For this review, take the finished solid that the model builds, in its own axes (mm). Give positions to 0.01 mm unless a question says otherwise; leave off trailing zeros. Loops run counter-clockwise (first coordinate to the right, second up) from the corner with the lowest first, then second, coordinate; pieces in that order, holes last. Notation, with made-up numbers: (57.25, 41) - (103.25, 41) arc R23 cw to (103.25, 75) - close; hole circle Ø2 at (-14, 15). An arc over 180 degrees is marked (long way). Answer in a Markdown table with one row per item.
```python
from build123d import *

# Parameters (mm, degrees)
CROQUIS1_W              = 50
CROQUIS1_H              = 55
CROQUIS1_R              = 3
SALIENTE_EXTRUIR1_DEPTH = 2.9
REDONDEO1_R             = 2
REDONDEO2_R             = 2


with BuildPart() as part:
    # Croquis1 → Saliente-Extruir1 (new body)
    with BuildSketch(Plane.XY):
        with Locations((25, 27.5)):
            Rectangle(CROQUIS1_W, CROQUIS1_H)
        with Locations((30, 42.5)):
            Circle(CROQUIS1_R, mode=Mode.SUBTRACT)
    extrude(amount=SALIENTE_EXTRUIR1_DEPTH)

    # Redondeo1
    redondeo1_edges = [part.edges().sort_by_distance(p)[0] for p in [
        (50, 0, 1.45),
        (0, 0, 1.45),
    ]]
    fillet(redondeo1_edges, radius=REDONDEO1_R)

    # Redondeo2
    redondeo2_edges = [part.edges().sort_by_distance(p)[0] for p in [
        (0, 55, 1.45),
        (50, 55, 1.45),
    ]]
    fillet(redondeo2_edges, radius=REDONDEO2_R)


solid = part.part
```
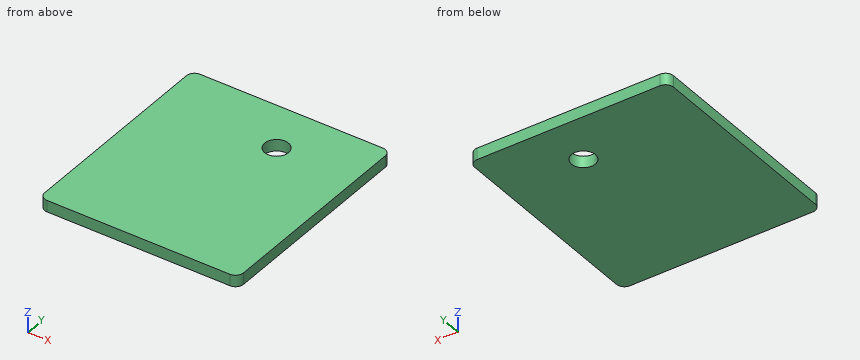
1. Clearance check with a flat-ended pin moving along its axis: pin 1 (3.5 mm diameter, centred on x = 30, y = 42.5, fed in from +Z). State where the tip first meets the part, or that it passes through.
Values:
| item | result |
|---|---|
| pin 1 | passes through |
2. Wall thickness on line 1 (Y direction, x = 30, z = 2.3): over which ranges is the line inside the solid? List them lowest first. Write a range as [from, to].
Values:
| item | result |
|---|---|
| line 1 | y = [0, 39.5], [45.5, 55] |
3. We need section A-A, the plane y = 42.5. Give the boundary of the cut face in (x, z), and give its area (3 significant figures).
Values:
| item | result |
|---|---|
| outline | (0, 0) - (27, 0) - (27, 2.9) - (0, 2.9) - close; (33, 0) - (50, 0) - (50, 2.9) - (33, 2.9) - close |
| area | 128 mm^2 |
4. We need section B-B, the plane x = 30. Give the boundary of the cut face in (y, z), and give its area (3 significant figures).
Values:
| item | result |
|---|---|
| outline | (0, 0) - (39.5, 0) - (39.5, 2.9) - (0, 2.9) - close; (45.5, 0) - (55, 0) - (55, 2.9) - (45.5, 2.9) - close |
| area | 142 mm^2 |
